Read the model definition and answer for the solid it produces. Units are mm, in the model's axes. A direction names the side the tool comes from. Coordinates: 2 decimals unless noted, no trailing zeros. Write each loop counter-clockwise with the first axis right and the second up, starting at its lowest first coordinate (ties: lowest second). Pieces come first, ordered by that corner, then holes.
(1) Section A-A on y = -2.7 is taken. Write down the section's boundary in (x, z).
(2) Section B-B on z = -3.5 is taken. Write down the section's boundary in (x, y), then the cut area to 3 significant figures.
(3) Section C-C on x = -6 is taken. Write down the section's boundary in (y, z), then the cut area to 3 significant figures.
(4) Which of the six approach directions +Z, -Z, +X, -X, +Y, -Y give full straight-line access (tool end or side, diameter ignored) to faces 5 (the flat face through (19, -2, -47.044)), 6 (the flat face through (-45, -2, -49.844)), 7 (the cylindrical face through (2.592, -1.622, -27.458)), 8 (the flat face through (19, -2, -49.844)), 9 (the flat face through (-42.533, -2, 16))?
(5) The mould has two halves that part along Z. Classify faces 1 (the flat face through (-28, -2, 77.956)), 2 (the flat face through (-13, -2, -52.044)), 3 (the cylindrical face through (-25.71, -1.62, -27.96)), 4 (the flat face through (21.801, -2, -48)): +Z half, -Z half, draft (parallel to the pull), parting line (faces both ways), or undercut.
(6) Find the intervals of material crossed by probe 1 along X at (y, z) = (-0.2, -30); probe 2 along X at (y, z) = (-2.3, -8); probe 3 along Z at (x, y) = (-40, -0.85), in increasing order.
(7) Given pin 1 (8 mm diameter, centred on x = -7, z = 49, fed in from +Y); pin 2 (1.5 mm diameter, centred on y = -2, z = 42.5, fed in from -X); pin 3 (0.7 mm diameter, centred on y = -2, z = -50.5, fed in from +X), each flat-ended and moving along its own axis, determine where each tip first touches the part or whether it passes through.
from build123d import *

# Parameters (mm, degrees)
F0_R      = 1.6
F0_W      = 30
F0_H      = 47.428162
F0_W_2    = 59.333406
F0_H_2    = 55.571838
F1_DEPTH  = 3.2
F2_DEPTH  = 2.3
F3_R      = 1.6
F4_DEPTH  = 11
F5_R      = 1.6
F6_DEPTH  = 11
F7_W      = 3.2
F7_H      = 2.8
F8_DEPTH  = 5
F9_W      = 3.2
F9_H      = 2.8
F10_DEPTH = 5
F11_R     = 1.6
F12_DEPTH = 8
F13_R     = 1.6
F14_DEPTH = 10


with BuildPart() as f1:
    # F0 (on Front) → F1 (new body)
    with BuildSketch(Plane.XZ):
        Polygon((-42.532899, 30.527938), (-42.532899, 3.527938), (16.800507, 3.527938), (-12.532899, 77.9561), (-12.532899, 30.527938), align=None)
        with Locations((-35.932899, 12.05425)):
            Circle(F0_R, mode=Mode.SUBTRACT)
        with Locations((-27.532899, 54.242019)):
            Rectangle(F0_W, F0_H)
        with Locations((-12.866196, -24.257981)):
            Rectangle(F0_W_2, F0_H_2)
    extrude(amount=F1_DEPTH)

    # F0 (on Front) → F2 (join)
    with BuildSketch(Plane.XZ):
        Polygon((-42.532899, 30.527938), (-42.532899, 3.527938), (16.800507, 3.527938), (-12.532899, 77.9561), (-12.532899, 30.527938), align=None)
        with Locations((-35.932899, 12.05425)):
            Circle(F0_R, mode=Mode.SUBTRACT)
        with Locations((-12.866196, -24.257981)):
            Rectangle(F0_W_2, F0_H_2)
        with Locations((-27.532899, 54.242019)):
            Rectangle(F0_W, F0_H)
    extrude(amount=F2_DEPTH)

    # F3 (on face) → F4 (cut)
    with BuildSketch(Plane.XZ.offset(3.2)):
        with Locations((11.800507, -25.4439)):
            Circle(F3_R)
    extrude(amount=-F4_DEPTH, mode=Mode.SUBTRACT)

    # F5 (on face) → F6 (cut)
    with BuildSketch(Plane.XZ.offset(3.2)):
        with Locations((-38.532899, 72.9561)):
            Circle(F5_R)
    extrude(amount=-F6_DEPTH, mode=Mode.SUBTRACT)

    # F7 (on face) → F8 (join)
    with BuildSketch(Plane.YZ.offset(16.800507)):
        with Locations((-1.6, -48.4439)):
            Rectangle(F7_W, F7_H)
    extrude(amount=F8_DEPTH)

    # F9 (on face) → F10 (join)
    with BuildSketch(Plane(origin=(-42.532899, 0, 0), x_dir=(0, -1, 0), z_dir=(-1, 0, 0))):
        with Locations((1.6, -48.4439)):
            Rectangle(F9_W, F9_H)
    extrude(amount=F10_DEPTH)

    # F11 (on face) → F12 (cut)
    with BuildSketch(Plane.XZ.offset(3.2)):
        with Locations((-24.532899, -29.0439)):
            Circle(F11_R)
    extrude(amount=-F12_DEPTH, mode=Mode.SUBTRACT)

    # F13 (on face) → F14 (cut)
    with BuildSketch(Plane.XZ.offset(3.2)):
        with Locations((2.800507, -29.0439)):
            Circle(F13_R)
    extrude(amount=-F14_DEPTH, mode=Mode.SUBTRACT)


solid = f1.part
Response:
1. outline: (-47.53, -49.84) - (-42.53, -49.84) - (-42.53, -52.04) - (16.8, -52.04) - (16.8, -49.84) - (21.8, -49.84) - (21.8, -47.04) - (16.8, -47.04) - (16.8, 3.53) - (-12.53, 77.96) - (-42.53, 77.96) - (-42.53, -47.04) - (-47.53, -47.04) - close; hole circle Ø3.2 at (-38.53, 72.96); hole circle Ø3.2 at (-35.93, 12.05); hole circle Ø3.2 at (-24.53, -29.04); hole circle Ø3.2 at (2.8, -29.04); hole circle Ø3.2 at (11.8, -25.44)
2. outline: (-42.53, -3.2) - (16.8, -3.2) - (16.8, 0) - (-42.53, 0) - close
2. area: 190 mm2
3. outline: (-3.2, -52.04) - (0, -52.04) - (0, 61.38) - (-3.2, 61.38) - close
3. area: 363 mm2
4. face 5: +Z, +X, +Y, -Y
4. face 6: -Z, -X, +Y, -Y
4. face 7: +Y, -Y
4. face 8: -Z, +X, +Y, -Y
4. face 9: +Z, -X, +Y, -Y
5. face 1: +Z half
5. face 2: -Z half
5. face 3: undercut
5. face 4: draft
6. probe 1: x = -42.53 to -25.82, -23.25 to 1.52, 4.08 to 16.8
6. probe 2: x = -42.53 to 16.8
6. probe 3: z = -52.04 to 72.32, 73.59 to 77.96
7. pin 1: stops at y = 0
7. pin 2: stops at x = -42.53
7. pin 3: stops at x = 16.8
